Design review of the part built by this model. Coordinates are the model's own, in mm. A direction names the side the tool comes from. Coordinates: 2 decimals unless noted, no trailing zeros. Answer as a JSON object with one key per item and string values. Group by question number.
1. Insertion check: pin 1 (0.6 mm diameter, centred on y = 14.5, z = 119, fed in from -X); pin 2 (1.2 mm diameter, centred on x = 14.5, z = 75, fed in from +Y); pin 3 (1.2 mm diameter, centred on x = 14, z = 150, fed in from -Y). Each pin has a flat end and moves straight along its axis. Give the tip position at first contact, or say it passes through.
2. Draft analysis for pull direction Y (two halves, no side actions). For faces 3 (the flat face through (15, 8, 133)), 4 (the flat face through (9.66, -8.39, 133.11)), 5 (the flat face through (-9.72, -8.45, 133.11)), 6 (the flat face through (-8, -15, 133)), state which applies: +Y half, -Y half, draft (parallel to the pull), parting line (faces both ways), or undercut.
3. To check wall thickness, follow probe 1 along Y at (x, z) = (5.75, 73); probe 2 along X at (y, z) = (4.75, 234); probe 3 along Y at (x, z) = (0.5, 80). State the ranges of each line that lie inside material, in increasing order.
4. Machinability: for faces 1 (the flat face through (0, -7.3, 133)), 2 (the flat face through (0, 7, 270)), which of the approach directions +Z, -Z, +X, -X, +Y, -Y give a long, thin tool a straight path to every point of the face, cutting with its end or side? Answer none if there is none.
from build123d import *

# Parameters (mm, degrees)
EXTRUDE1_DEPTH = 270


with BuildPart() as part:
    # Sketch1 → Extrude1 (new body)
    with BuildSketch(Plane.XY):
        with BuildLine():
            Line((-12, 15), (-4.3, 15))
            ThreePointArc((-4.3, 15), (-4.158578644, 14.941421356), (-4.1, 14.8))
            Line((-4.1, 14.8), (-4.1, 13.7))
            ThreePointArc((-4.1, 13.7), (-4.158578644, 13.558578644), (-4.3, 13.5))
            Line((-4.3, 13.5), (-9.812994231, 13.5))
            ThreePointArc((-9.812994231, 13.5), (-10.736873764, 12.882683432), (-10.520101013, 11.792893219))
            Line((-10.520101013, 11.792893219), (-6.320101013, 7.592893219))
            ThreePointArc((-6.320101013, 7.592893219), (-5.995677664, 7.376120467), (-5.612994231, 7.3))
            Line((-5.612994231, 7.3), (5.612994231, 7.3))
            ThreePointArc((5.612994231, 7.3), (5.995677664, 7.376120467), (6.320101013, 7.592893219))
            Line((6.320101013, 7.592893219), (10.520101013, 11.792893219))
            ThreePointArc((10.520101013, 11.792893219), (10.736873764, 12.882683432), (9.812994231, 13.5))
            Line((9.812994231, 13.5), (4.3, 13.5))
            ThreePointArc((4.3, 13.5), (4.158578644, 13.558578644), (4.1, 13.7))
            Line((4.1, 13.7), (4.1, 14.8))
            ThreePointArc((4.1, 14.8), (4.158578644, 14.941421356), (4.3, 15))
            Line((4.3, 15), (12, 15))
            ThreePointArc((12, 15), (14.121320344, 14.121320344), (15, 12))
            Line((15, 12), (15, 4.3))
            ThreePointArc((15, 4.3), (14.941421356, 4.158578644), (14.8, 4.1))
            Line((14.8, 4.1), (13.7, 4.1))
            ThreePointArc((13.7, 4.1), (13.558578644, 4.158578644), (13.5, 4.3))
            Line((13.5, 4.3), (13.5, 9.812994231))
            ThreePointArc((13.5, 9.812994231), (12.882683432, 10.736873764), (11.792893219, 10.520101013))
            Line((11.792893219, 10.520101013), (7.592893219, 6.320101013))
            ThreePointArc((7.592893219, 6.320101013), (7.376120467, 5.995677664), (7.3, 5.612994231))
            Line((7.3, 5.612994231), (7.3, -5.612994231))
            ThreePointArc((7.3, -5.612994231), (7.376120467, -5.995677664), (7.592893219, -6.320101013))
            Line((7.592893219, -6.320101013), (11.792893219, -10.520101013))
            ThreePointArc((11.792893219, -10.520101013), (12.882683432, -10.736873764), (13.5, -9.812994231))
            Line((13.5, -9.812994231), (13.5, -4.3))
            ThreePointArc((13.5, -4.3), (13.558578644, -4.158578644), (13.7, -4.1))
            Line((13.7, -4.1), (14.8, -4.1))
            ThreePointArc((14.8, -4.1), (14.941421356, -4.158578644), (15, -4.3))
            Line((15, -4.3), (15, -12))
            ThreePointArc((15, -12), (14.121320344, -14.121320344), (12, -15))
            Line((12, -15), (4.3, -15))
            ThreePointArc((4.3, -15), (4.158578644, -14.941421356), (4.1, -14.8))
            Line((4.1, -14.8), (4.1, -13.7))
            ThreePointArc((4.1, -13.7), (4.158578644, -13.558578644), (4.3, -13.5))
            Line((4.3, -13.5), (9.812994231, -13.5))
            ThreePointArc((9.812994231, -13.5), (10.736873764, -12.882683432), (10.520101013, -11.792893219))
            Line((10.520101013, -11.792893219), (6.320101013, -7.592893219))
            ThreePointArc((6.320101013, -7.592893219), (5.995677664, -7.376120467), (5.612994231, -7.3))
            Line((5.612994231, -7.3), (-5.612994231, -7.3))
            ThreePointArc((-5.612994231, -7.3), (-5.995677664, -7.376120467), (-6.320101013, -7.592893219))
            Line((-6.320101013, -7.592893219), (-10.520101013, -11.792893219))
            ThreePointArc((-10.520101013, -11.792893219), (-10.736873764, -12.882683432), (-9.812994231, -13.5))
            Line((-9.812994231, -13.5), (-4.3, -13.5))
            ThreePointArc((-4.3, -13.5), (-4.158578644, -13.558578644), (-4.1, -13.7))
            Line((-4.1, -13.7), (-4.1, -14.8))
            ThreePointArc((-4.1, -14.8), (-4.158578644, -14.941421356), (-4.3, -15))
            Line((-4.3, -15), (-12, -15))
            ThreePointArc((-12, -15), (-14.121320344, -14.121320344), (-15, -12))
            Line((-15, -12), (-15, -4.3))
            ThreePointArc((-15, -4.3), (-14.941421356, -4.158578644), (-14.8, -4.1))
            Line((-14.8, -4.1), (-13.7, -4.1))
            ThreePointArc((-13.7, -4.1), (-13.558578644, -4.158578644), (-13.5, -4.3))
            Line((-13.5, -4.3), (-13.5, -9.812994231))
            ThreePointArc((-13.5, -9.812994231), (-12.882683432, -10.736873764), (-11.792893219, -10.520101013))
            Line((-11.792893219, -10.520101013), (-7.592893219, -6.320101013))
            ThreePointArc((-7.592893219, -6.320101013), (-7.376120467, -5.995677664), (-7.3, -5.612994231))
            Line((-7.3, -5.612994231), (-7.3, 5.612994231))
            ThreePointArc((-7.3, 5.612994231), (-7.376120467, 5.995677664), (-7.592893219, 6.320101013))
            Line((-7.592893219, 6.320101013), (-11.792893219, 10.520101013))
            ThreePointArc((-11.792893219, 10.520101013), (-12.882683432, 10.736873764), (-13.5, 9.812994231))
            Line((-13.5, 9.812994231), (-13.5, 4.3))
            ThreePointArc((-13.5, 4.3), (-13.558578644, 4.158578644), (-13.7, 4.1))
            Line((-13.7, 4.1), (-14.8, 4.1))
            ThreePointArc((-14.8, 4.1), (-14.941421356, 4.158578644), (-15, 4.3))
            Line((-15, 4.3), (-15, 12))
            ThreePointArc((-15, 12), (-14.121320344, 14.121320344), (-12, 15))
        make_face()
        with BuildLine():
            Line((-3.04762381, 4.744680085), (-2.445405681, 4.142461956))
            ThreePointArc((-2.445405681, 4.142461956), (-2.06276965, 3.937478186), (-1.630658427, 3.978813026))
            ThreePointArc((-1.630658427, 3.978813026), (0, 4.3), (1.630658427, 3.978813026))
            ThreePointArc((1.630658427, 3.978813026), (2.06276965, 3.937478186), (2.445405681, 4.142461956))
            Line((2.445405681, 4.142461956), (3.04762381, 4.744680085))
            ThreePointArc((3.04762381, 4.744680085), (3.171115834, 4.802453455), (3.302939637, 4.767660826))
            ThreePointArc((3.302939637, 4.767660826), (4.101219331, 4.101219331), (4.767660826, 3.302939637))
            ThreePointArc((4.767660826, 3.302939637), (4.802453455, 3.171115834), (4.744680085, 3.04762381))
            Line((4.744680085, 3.04762381), (4.142461956, 2.445405681))
            ThreePointArc((4.142461956, 2.445405681), (3.937478186, 2.06276965), (3.978813026, 1.630658427))
            ThreePointArc((3.978813026, 1.630658427), (4.3, 0), (3.978813026, -1.630658427))
            ThreePointArc((3.978813026, -1.630658427), (3.937478186, -2.06276965), (4.142461956, -2.445405681))
            Line((4.142461956, -2.445405681), (4.744680085, -3.04762381))
            ThreePointArc((4.744680085, -3.04762381), (4.802453455, -3.171115834), (4.767660826, -3.302939637))
            ThreePointArc((4.767660826, -3.302939637), (4.101219331, -4.101219331), (3.302939637, -4.767660826))
            ThreePointArc((3.302939637, -4.767660826), (3.171115834, -4.802453455), (3.04762381, -4.744680085))
            Line((3.04762381, -4.744680085), (2.445405681, -4.142461956))
            ThreePointArc((2.445405681, -4.142461956), (2.06276965, -3.937478186), (1.630658427, -3.978813026))
            ThreePointArc((1.630658427, -3.978813026), (0, -4.3), (-1.630658427, -3.978813026))
            ThreePointArc((-1.630658427, -3.978813026), (-2.06276965, -3.937478186), (-2.445405681, -4.142461956))
            Line((-2.445405681, -4.142461956), (-3.04762381, -4.744680085))
            ThreePointArc((-3.04762381, -4.744680085), (-3.171115834, -4.802453455), (-3.302939637, -4.767660826))
            ThreePointArc((-3.302939637, -4.767660826), (-4.101219331, -4.101219331), (-4.767660826, -3.302939637))
            ThreePointArc((-4.767660826, -3.302939637), (-4.802453455, -3.171115834), (-4.744680085, -3.04762381))
            Line((-4.744680085, -3.04762381), (-4.142461956, -2.445405681))
            ThreePointArc((-4.142461956, -2.445405681), (-3.937478186, -2.06276965), (-3.978813026, -1.630658427))
            ThreePointArc((-3.978813026, -1.630658427), (-4.3, 0), (-3.978813026, 1.630658427))
            ThreePointArc((-3.978813026, 1.630658427), (-3.937478186, 2.06276965), (-4.142461956, 2.445405681))
            Line((-4.142461956, 2.445405681), (-4.744680085, 3.04762381))
            ThreePointArc((-4.744680085, 3.04762381), (-4.802453455, 3.171115834), (-4.767660826, 3.302939637))
            ThreePointArc((-4.767660826, 3.302939637), (-4.101219331, 4.101219331), (-3.302939637, 4.767660826))
            ThreePointArc((-3.302939637, 4.767660826), (-3.171115834, 4.802453455), (-3.04762381, 4.744680085))
        make_face(mode=Mode.SUBTRACT)
    extrude(amount=EXTRUDE1_DEPTH)


solid = part.part
Findings below:
{
 "1": {"pin 1": "stops at x = -14.04", "pin 2": "stops at y = 14.32", "pin 3": "stops at y = -14.65"},
 "2": {"face 3": "draft", "face 4": "undercut", "face 5": "undercut", "face 6": "-Y half"},
 "3": {"probe 1": "y = -15 to -13.5, -7.31 to 7.31, 13.5 to 15", "probe 2": "x = -15 to -13.5, -7.3 to -3.33, -3.05 to 3.05, 3.33 to 7.3, 13.5 to 15", "probe 3": "y = -7.3 to -4.27, 4.27 to 7.3"},
 "4": {"face 1": "+Z, -Z", "face 2": "+Z, +X, -X, +Y, -Y"}
}
